Can you work these out from the drawing? Everything is in mm from the part's minimum corner. A direction names the side the tool comes from. Give positions to 0.01 mm unless a question says otherwise; leave off trailing zeros. Loops run counter-clockwise (first coordinate to the right, second up) from the corner with the lowest first, then second, coordinate; pieces in that order, holes last. Notation, with made-up numbers: (58.5, 61) - (109.5, 61) arc R8 ccw to (109.5, 73) - close; hole circle Ø3 at (31, -22.5). An arc over 180 degrees is marked (long way). One line per item, written item: value. Start each with the question number.
Q1. I'm going to push flat-ended pins straight in: P1, Ø9, axis at x = 10, y = 12, coming from the -Z side; P2, Ø12, axis at x = 84.5, y = 34.5, coming from the +Z side; P3, Ø9, axis at x = 53.5, y = 17.5, coming from the -Z side; P4, Ø9, axis at y = 19, z = 39, coming from the +X side. Where does each tip first touch, or does it pass through?
Q2. If I drill on line 1 (X direction, y = 11, z = 26.5); line 2 (Y direction, x = 86, z = 2); line 3 (Z direction, x = 88, y = 24), over which ranges is the centre line in solid material (lowest first)? Write a range as from..to.
Q3. I want a section at A-A (x = 86.5). Please give me the cut outline in (y, z).
Q4. I want a section at D-D (x = 48). Please give me the cut outline in (y, z).
Q5. I want a section at C-C (y = 25.5). Please give me the cut outline in (x, z), then the cut area to 3 significant figures.
Q6. For the marked faces 1, 2 and 3, which set-ups out of +Z, -Z, +X, -X, +Y, -Y let a thin tool reach every point of the face, with its end or its side?
Q7. I want a section at B-B (z = 47). Please give me the cut outline in (x, y).
Q8. If we mould it in two halves opening along Y, with no side actions, what happens to the marked faces 4, 5, 6 and 7? For each: released by +Y, released by -Y, zero draft, split by the parting line, or undercut.
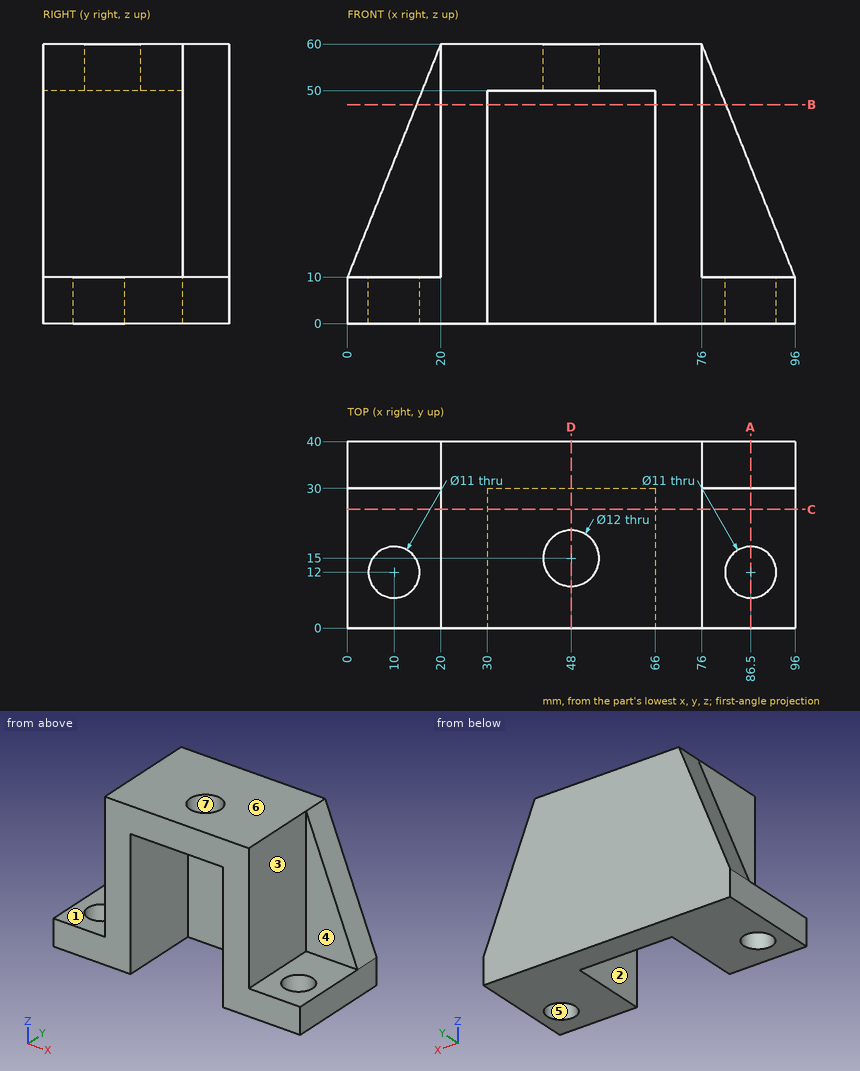
Worked answers:
1. P1: passes through
1. P2: stops at z = 53.75
1. P3: stops at z = 50
1. P4: stops at x = 76
2. line 1: x = 20..30, 66..76
2. line 2: y = 0..6.52, 17.48..40
2. line 3: z = 0..10
3. outline: (0, 0) - (6.5, 0) - (6.5, 10) - (0, 10) - close; (17.5, 0) - (40, 0) - (40, 33.75) - (30, 33.75) - (30, 10) - (17.5, 10) - close
4. outline: (0, 50) - (9, 50) - (9, 60) - (0, 60) - close; (21, 50) - (30, 50) - (30, 0) - (40, 0) - (40, 60) - (21, 60) - close
5. outline: (0, 0) - (30, 0) - (30, 50) - (66, 50) - (66, 0) - (96, 0) - (96, 10) - (76, 10) - (76, 60) - (20, 60) - (20, 10) - (0, 10) - close
5. area: 1,960 mm²
6. face 1: +Z, -X, -Y
6. face 2: -Z, -Y
6. face 3: +Z, +X, -Y
7. outline: (14.8, 30) - (20, 30) - (20, 0) - (30, 0) - (30, 30) - (66, 30) - (66, 0) - (76, 0) - (76, 30) - (81.2, 30) - (81.2, 40) - (14.8, 40) - close
8. face 4: released by -Y
8. face 5: undercut
8. face 6: zero draft
8. face 7: undercut
